Here's how the part is built. I have some questions about the finished solid (model axes, mm). Coordinates: 2 decimals unless noted, no trailing zeros. Write each loop counter-clockwise with the first axis right and the second up, starting at its lowest first coordinate (ties: lowest second). Pieces come first, ordered by that corner, then holes.
Item 1: If I drill on line 1 (Y direction, x = 10.25, z = 273.05); line 2 (Y direction, x = 2, z = 6); line 3 (X direction, y = 2.25, z = 18.5), over which ranges is the centre line in solid material (lowest first)?
Item 2: I'm going to push flat-ended pins straight in: pin 1 Ø10 at (x, z) = (20, 127.5) entering from -Y; pin 2 Ø6 at (y, z) = (6.35, 6.35) entering from -X; pin 3 Ø1.5 at (x, y) = (39, 8) entering from +Z; pin 4 Ø4 at (y, z) = (11.5, 142) entering from +X. Where does each tip first touch, or does it pass through?
Item 3: If we section it at D-D (z = 94.5): Please give me the cut outline in (x, y).
Item 4: If we section it at A-A (z = 64): Please give me the cut outline in (x, y).
Item 5: If we section it at C-C (z = 232.5): Please give me the cut outline in (x, y).
Item 6: If we section it at B-B (x = 25.5): Please give me the cut outline in (y, z), then the cut area to 3 significant figures.
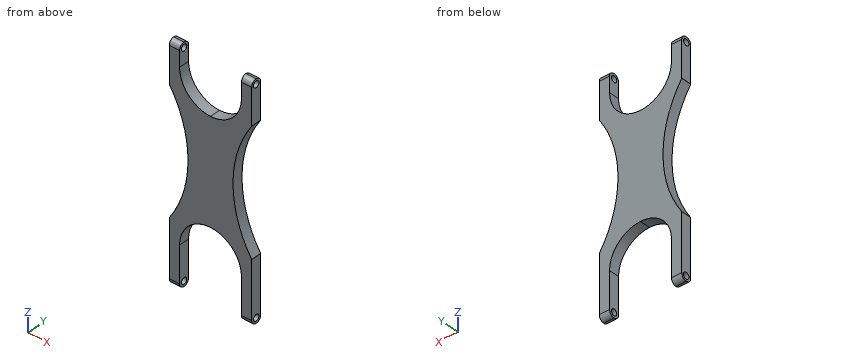
from build123d import *

# Parameters (mm, degrees)
BOSS_EXTRUDE1_DEPTH = 12.7
FILLET1_R           = 6.35
SKETCH2_R           = 3.81
CUT_EXTRUDE1_DEPTH  = 298.570512652
SKETCH3_R           = 3.81
CUT_EXTRUDE2_DEPTH  = 298.570512652


with BuildPart() as part:
    # Sketch1 → Boss-Extrude1 (new body)
    with BuildSketch(Plane(origin=(0, 0, 0), x_dir=(1, 0, 0), z_dir=(0, 1, 0))):
        with BuildLine():
            Line((0, 0), (12.7, 0))
            Line((12.7, 0), (12.7, -50.8))
            ThreePointArc((12.7, -50.8), (23.859231637, -77.740768363), (50.8, -88.9))
            ThreePointArc((50.8, -88.9), (77.740768363, -77.740768363), (88.9, -50.8))
            Line((88.9, -50.8), (88.9, 0))
            Line((88.9, 0), (101.6, 0))
            Line((101.6, 0), (101.6, -76.2))
            ThreePointArc((101.6, -76.2), (78.528496405, -152.4), (101.6, -228.6))
            Line((101.6, -228.6), (101.6, -279.4))
            Line((101.6, -279.4), (88.9, -279.4))
            Line((88.9, -279.4), (88.9, -254))
            ThreePointArc((88.9, -254), (77.740768363, -227.059231637), (50.8, -215.9))
            ThreePointArc((50.8, -215.9), (23.859231637, -227.059231637), (12.7, -254))
            Line((12.7, -254), (12.7, -279.4))
            Line((12.7, -279.4), (0, -279.4))
            Line((0, -279.4), (0, -228.6))
            ThreePointArc((0, -228.6), (23.071503595, -152.4), (0, -76.2))
            Line((0, -76.2), (0, 0))
        make_face()
    extrude(amount=BOSS_EXTRUDE1_DEPTH)

    # Fillet1
    fillet1_edges = [part.edges().sort_by_distance(p)[0] for p in [
        (95.25, 0, 0),
        (6.35, 0, 0),
        (95.25, 12.7, 0),
        (6.35, 12.7, 0),
        (6.35, 0, 279.4),
        (6.35, 12.7, 279.4),
        (95.25, 0, 279.4),
        (95.25, 12.7, 279.4),
    ]]
    fillet(fillet1_edges, radius=FILLET1_R - 0.0001)  # a hair under: the kernel refuses the full size

    # Sketch2 → Cut-Extrude1 (cut, through all)
    with BuildSketch(Plane(origin=(101.6, 0, 0), x_dir=(0, 0, -1), z_dir=(1, 0, 0))):
        with Locations((-273.05, 6.35)):
            Circle(SKETCH2_R)
    extrude(amount=-CUT_EXTRUDE1_DEPTH, mode=Mode.SUBTRACT)

    # Sketch3 → Cut-Extrude2 (cut, through all)
    with BuildSketch(Plane(origin=(101.6, 0, 0), x_dir=(0, 0, -1), z_dir=(1, 0, 0))):
        with Locations((-6.35, 6.35)):
            Circle(SKETCH3_R)
    extrude(amount=-CUT_EXTRUDE2_DEPTH, mode=Mode.SUBTRACT)


solid = part.part
Answer list:
1. line 1: y = 0 to 2.54, 10.16 to 12.7
1. line 2: y = 0.01 to 2.56, 10.14 to 12.69
1. line 3: x = 0 to 12.7, 88.9 to 101.6
2. pin 1: stops at y = 0
2. pin 2: passes through
2. pin 3: stops at z = 218.03
2. pin 4: stops at x = 79.09
3. outline: (10.27, 0) - (91.33, 0) - (91.33, 12.7) - (10.27, 12.7) - close
4. outline: (0, 0) - (15.06, 0) - (15.06, 12.7) - (0, 12.7) - close; (86.54, 0) - (101.6, 0) - (101.6, 12.7) - (86.54, 12.7) - close
5. outline: (0, 0) - (19.35, 0) - (19.35, 12.7) - (0, 12.7) - close; (82.25, 0) - (101.6, 0) - (101.6, 12.7) - (82.25, 12.7) - close
6. outline: (0, 79.29) - (12.7, 79.29) - (12.7, 225.51) - (0, 225.51) - close
6. area: 1,860 mm2
